Here's how the part is built. I have some questions about the finished solid (model axes, mm). A direction names the side the tool comes from. Give positions to 0.01 mm unless a question says otherwise; leave off trailing zeros. Write each loop counter-clockwise with the first axis right and the second up, starting at its lowest first coordinate (ties: lowest second). Pieces come first, ordered by that corner, then holes. Notation, with made-up numbers: (29, 53.25) -> (33, 53.25) arc R22 ccw to (33, 70.25) -> close; hole circle Ø7 at (35, 49). An arc over 180 degrees is marked (long way). Return JSON: item names as keys, results as strings.
from build123d import *

# Parameters (mm, degrees)
BOSS_EXTRUDE1_DEPTH = 300
CUT_EXTRUDE1_DEPTH  = 274.6


with BuildPart() as part:
    # Sketch1 → Boss-Extrude1 (new body)
    with BuildSketch(Plane(origin=(0, 0, 0), x_dir=(1, 0, 0), z_dir=(0, 1, 0))):
        Polygon((359.6, 1066.8), (-359.6, 1066.8), (-359.6, 566.8), (359.6, 566.8), (359.6, 0), (859.6, 0), (859.6, 1066.8), align=None)
    extrude(amount=BOSS_EXTRUDE1_DEPTH)

    # Sketch2 → Cut-Extrude1 (cut)
    with BuildSketch(Plane(origin=(0, 300, 0), x_dir=(1, 0, 0), z_dir=(0, 1, 0))):
        Polygon((834.2, 25.4), (834.2, 1041.4), (-334.2, 1041.4), (-334.2, 592.2), (385, 592.2), (385, 25.4), align=None)
    extrude(amount=-CUT_EXTRUDE1_DEPTH, mode=Mode.SUBTRACT)


solid = part.part
1. If we mould it in two halves opening along X, with no side actions, what happens to faces 1 (the face through (606, 148, 0)), 2 (the face through (-359.6, 148, -820)), 3 (the face through (834.2, 165, -526))? For each: released by +X, released by -X, zero draft, split by the parting line, or undercut.
Taken from the geometry:
{"face 1": "zero draft", "face 2": "released by -X", "face 3": "undercut"}
2. Suppose I cut it at B-B, the plane x = 0. List the corners of the cut face in (y, z) for me, and give its area (3 significant figures).
Taken from the geometry:
{"outline": "(0, -1066.8) -> (300, -1066.8) -> (300, -1041.4) -> (25.4, -1041.4) -> (25.4, -592.2) -> (300, -592.2) -> (300, -566.8) -> (0, -566.8) -> close", "area": "26,600 mm²"}
3. If I drill on line 1 (X direction, y = 267.5, z = -279); line 2 (X direction, y = 74.5, z = -749); line 3 (Z direction, x = 409.5, y = 193), over which ranges is the centre line in solid material (lowest first)? Write a range as [from, to].
Taken from the geometry:
{"line 1": "x = [359.6, 385], [834.2, 859.6]", "line 2": "x = [-359.6, -334.2], [834.2, 859.6]", "line 3": "z = [-1066.8, -1041.4], [-25.4, 0]"}
4. Suppose I cut it at A-A, the plane y = 145.5. List the corners of the cut face in (x, z) for me, and give its area (3 significant figures).
Taken from the geometry:
{"outline": "(-359.6, -1066.8) -> (859.6, -1066.8) -> (859.6, 0) -> (359.6, 0) -> (359.6, -566.8) -> (-359.6, -566.8) -> close; hole (-334.2, -1041.4) -> (834.2, -1041.4) -> (834.2, -25.4) -> (385, -25.4) -> (385, -592.2) -> (-334.2, -592.2) -> close", "area": "114,000 mm²"}
5. Suppose I cut it at C-C, the plane z = -70.5. List the corners of the cut face in (x, y) for me, and give its area (3 significant figures).
Taken from the geometry:
{"outline": "(359.6, 0) -> (859.6, 0) -> (859.6, 300) -> (834.2, 300) -> (834.2, 25.4) -> (385, 25.4) -> (385, 300) -> (359.6, 300) -> close", "area": "26,600 mm²"}
6. For pin 1 Ø4 at (y, z) = (172.5, -338) entering from -X; pin 2 Ø5 at (x, y) = (50.5, 192.5) entering from +Z, each with a flat end and sliding along its axis, tell me the tip position at first contact or that it passes through.
Taken from the geometry:
{"pin 1": "stops at x = 359.6", "pin 2": "stops at z = -566.8"}
7. Which directions (+Z, -Z, +X, -X, +Y, -Y) give clear straight access to the entire face, cutting with the end or side of a thin tool? Please do faces 4 (the face through (-5, 148, -566.8)), 5 (the face through (606, 165, -25.4)), 6 (the face through (859.6, 148, -526)).
Taken from the geometry:
{"face 4": "+Z, -X, +Y, -Y", "face 5": "+Y", "face 6": "+Z, -Z, +X, +Y, -Y"}
